Geometry: final body of the model. Coordinates: model frame, mm. A direction names the side the tool comes from. Give positions to 0.01 mm unless a question says otherwise; leave off trailing zeros. Loops run counter-clockwise (first coordinate to the right, second up) from the corner with the lowest first, then second, coordinate; pieces in that order, holes last. Notation, with made-up numbers: M -3.5,5.5 L 33.5,5.5 A18 ccw 33.5,25.5 Z; hole C 12,68.5 d3. An arc over 180 degrees is marked long. One line per question, with ' | ' between items. Start each with the question number.
from build123d import *

# Parameters (mm, degrees)
CROQUIS1_R              = 55
CROQUIS1_W              = 45
CROQUIS1_H              = 15
SALIENTE_EXTRUIR1_DEPTH = 10
CROQUIS2_W              = 10
CROQUIS2_H              = 30
SALIENTE_EXTRUIR2_DEPTH = 65
CROQUIS3_R              = 1.5
CORTAR_EXTRUIR1_DEPTH   = 50
CORTAR_EXTRUIR2_DEPTH   = 10
CROQUIS5_R              = 2.5
CORTAR_EXTRUIR3_DEPTH   = 85
CROQUIS8_R              = 1.5
CORTAR_EXTRUIR4_DEPTH   = 10
CROQUIS10_R             = 2.575
CROQUIS11_W             = 10
CROQUIS11_H             = 70
CORTAR_EXTRUIR5_DEPTH   = 30
CORTAR_EXTRUIR6_DEPTH   = 30
SALIENTE_EXTRUIR4_REACH = 80.422
CROQUIS13_W             = 10
CROQUIS13_H             = 30
CROQUIS7_R              = 1.5
CORTAR_EXTRUIR9_DEPTH   = 10


with BuildPart() as part:
    # Croquis1 → Saliente-Extruir1 (new body)
    with BuildSketch(Plane.XY):
        Circle(CROQUIS1_R)
        with Locations((0, -2.5)):
            Rectangle(CROQUIS1_W, CROQUIS1_H, mode=Mode.SUBTRACT)
    extrude(amount=SALIENTE_EXTRUIR1_DEPTH)

    # Croquis2 → Saliente-Extruir2 (add)
    with BuildSketch(Plane.XY.offset(10)):
        with Locations((30, 0)):
            Rectangle(CROQUIS2_W, CROQUIS2_H)
    extrude(amount=SALIENTE_EXTRUIR2_DEPTH)

    # Croquis3 → Cortar-Extruir1 (cut)
    with BuildSketch(Plane.XZ.offset(15)):
        with Locations((30, 70)):
            Circle(CROQUIS3_R)
    extrude(amount=-CORTAR_EXTRUIR1_DEPTH, mode=Mode.SUBTRACT)

    # Croquis4 → Cortar-Extruir2 (cut)
    with BuildSketch(Plane.XZ.offset(15)):
        Polygon((35, 65), (25, 42.602429787), (25, 65), (25, 75), (35, 75), align=None)
    cortar_extruir2 = extrude(amount=-CORTAR_EXTRUIR2_DEPTH, mode=Mode.SUBTRACT)

    # Simetría1: Cortar-Extruir2 across plane
    add(cortar_extruir2.mirror(Plane.ZX), mode=Mode.SUBTRACT)

    # Croquis5 → Cortar-Extruir3 (cut, symmetric)
    with BuildSketch(Plane.XZ.offset(-5)):
        with Locations(Location((0, 5, 0), (0, 0, 270))):
            Circle(CROQUIS5_R)
    extrude(amount=CORTAR_EXTRUIR3_DEPTH, both=True, mode=Mode.SUBTRACT)

    # Croquis8 → Cortar-Extruir4 (cut)
    with BuildSketch(Plane.XY.offset(10)):
        with Locations(Location((9.999999991, -33.6, 0), (0, 0, 180))):
            Circle(CROQUIS8_R)
        with Locations(Location((19.999999995, 25, 0), (0, 0, 180))):
            Circle(CROQUIS8_R)
        with Locations((-20.000000005, 25)):
            Circle(CROQUIS8_R)
        with Locations((-10, -33.6)):
            Circle(CROQUIS8_R)
    extrude(amount=-CORTAR_EXTRUIR4_DEPTH, mode=Mode.SUBTRACT)

    # Croquis10 → Cortar-Revolución1 (revolve, cut)
    with BuildSketch(Plane(origin=(0, 0, 0), x_dir=(1, 0, 0), z_dir=(0, 1, 0))):
        with Locations((-55, -5)):
            Circle(CROQUIS10_R)
    revolve(axis=Axis((0, 0, 0), (0, 0, 1)), mode=Mode.SUBTRACT)

    # Croquis11 → Cortar-Extruir5 (cut)
    with BuildSketch(Plane(origin=(0, 15, 0), x_dir=(1, 0, 0), z_dir=(0, 1, 0))):
        with Locations((30, -40)):
            Rectangle(CROQUIS11_W, CROQUIS11_H)
    extrude(amount=-CORTAR_EXTRUIR5_DEPTH, mode=Mode.SUBTRACT)

    # Croquis12 → Cortar-Extruir6 (cut)
    with BuildSketch(Plane.XZ.offset(-15)):
        Polygon((35, 10), (45, 10), (45, 5), (35, 5), (25, 5), (25, 10), align=None)
    extrude(amount=CORTAR_EXTRUIR6_DEPTH, mode=Mode.SUBTRACT)

    # Croquis13 → Saliente-Extruir4 (add, up to next)
    with BuildSketch(Plane.XY.offset(10), mode=Mode.PRIVATE) as saliente_extruir4_sk1:
        with Locations((30, 0)):
            Rectangle(CROQUIS13_W, CROQUIS13_H)
    saliente_extruir4_tool1 = extrude(saliente_extruir4_sk1.sketch, amount=-SALIENTE_EXTRUIR4_REACH, mode=Mode.PRIVATE) - part.part
    add(saliente_extruir4_tool1.solids().sort_by_distance((30, 0, 10))[0])

    # Croquis7 → Cortar-Extruir9 (cut)
    with BuildSketch(Plane.XY.offset(10)):
        with Locations((0, 41)):
            Circle(CROQUIS7_R)
    extrude(amount=-CORTAR_EXTRUIR9_DEPTH, mode=Mode.SUBTRACT)


solid = part.part
Q1. Section A-A, the plane y = 0. Output: boundary loops of the cut face in (x, z) (3 decimals), plus the area to 3 significant figures.
Q2. Draft query along Y for faces 4 (the flat face through (-1, -11, 10)), 5 (the cylindrical face through (25.379, -48.794, 8.771)), 6 (the flat face through (40, 0, 5)). Return one class per face: released by +Y, released by -Y, zero draft, split by the parting line, or undercut.
Q3. Section B-B, the plane x = 0. Output: boundary loops of the cut face in (y, z) (3 decimals), plus the area to 3 significant figures.
Q4. Set-up query: faces 1 (the flat face through (22.5, -3, 5)), 2 (the flat face through (35, 0, 8)), 3 (the flat face through (-1, -11, 0)). Return all of +Z, -Z, +X, -X, +Y, -Y with unobstructed straight access to the full face (end or side cutting, diameter ignored); none if empty.
Q5. Section C-C, the plane y = -33.6. Count the separate pieces of the cut face and the enclosed holes in it, plus the area to 3 significant figures.
Q6. Material intervals for L1, parallel to Y at x = 0, z = 8.35; L2, parallel to Y at x = -1, z = 2.25; L3, parallel to Z at x = 0, y = -21, sorted ascending.
Q7. Contact query for flat-ended pins moving along their axis: pin 1 (1.5 mm diameter, centred on x = 38, z = 8, fed in from -Y); pin 2 (1.5 mm diameter, centred on y = 24, z = 2, fed in from +X); pin 3 (3 mm diameter, centred on x = 6, z = 3.5, fed in from -Y). Output: stop coordinate, or through.
Model answer:
1) outline: M -55,0 L -22.5,0 L -22.5,10 L -55,10 L -55,7.575 A2.575 cw -55,2.425 Z; M 22.5,0 L 55,0 L 55,2.425 A2.575 cw 55,7.575 L 55,10 L 45,10 L 45,5 L 35,5 L 35,10 L 22.5,10 Z | area: 579 mm^2
2) face 4: zero draft | face 5: split by the parting line | face 6: undercut
3) outline: M -55,0 L -10,0 L -10,2.5 L -54.383,2.5 A2.575 cw -55,2.425 Z; M -55,7.575 A2.575 cw -54.383,7.5 L -10,7.5 L -10,10 L -55,10 Z; M 5,0 L 39.5,0 L 39.5,2.5 L 5,2.5 Z; M 5,7.5 L 39.5,7.5 L 39.5,10 L 5,10 Z; M 42.5,0 L 55,0 L 55,2.425 A2.575 cw 54.383,2.5 L 42.5,2.5 Z; M 42.5,7.5 L 54.383,7.5 A2.575 cw 55,7.575 L 55,10 L 42.5,10 Z | area: 460 mm^2
4) face 1: +Z, -Z | face 2: +Z | face 3: -Z, +X, -X, +Y, -Y
5) separate pieces: 3 | enclosed holes: 1 | area: 765 mm^2
6) L1: y = -55 to -10, 5 to 39.5, 42.5 to 55 | L2: y = -54.99 to -10, 5 to 39.88, 42.12 to 54.99 | L3: z = 0 to 2.5, 7.5 to 10
7) pin 1: stops at y = -40.47 | pin 2: stops at x = 49.84 | pin 3: stops at y = -54.78
